Answer from the drawing. Dimensions are ordinates in mm from the lowest x, y and z of the part. Give positions to 0.01 mm unless a question says otherwise; leave off trailing zeros. Write each loop counter-clockwise with the first axis right and the second up, starting at its lowest first coordinate (ties: lowest second). Pieces come first, ordered by that corner, then holes.
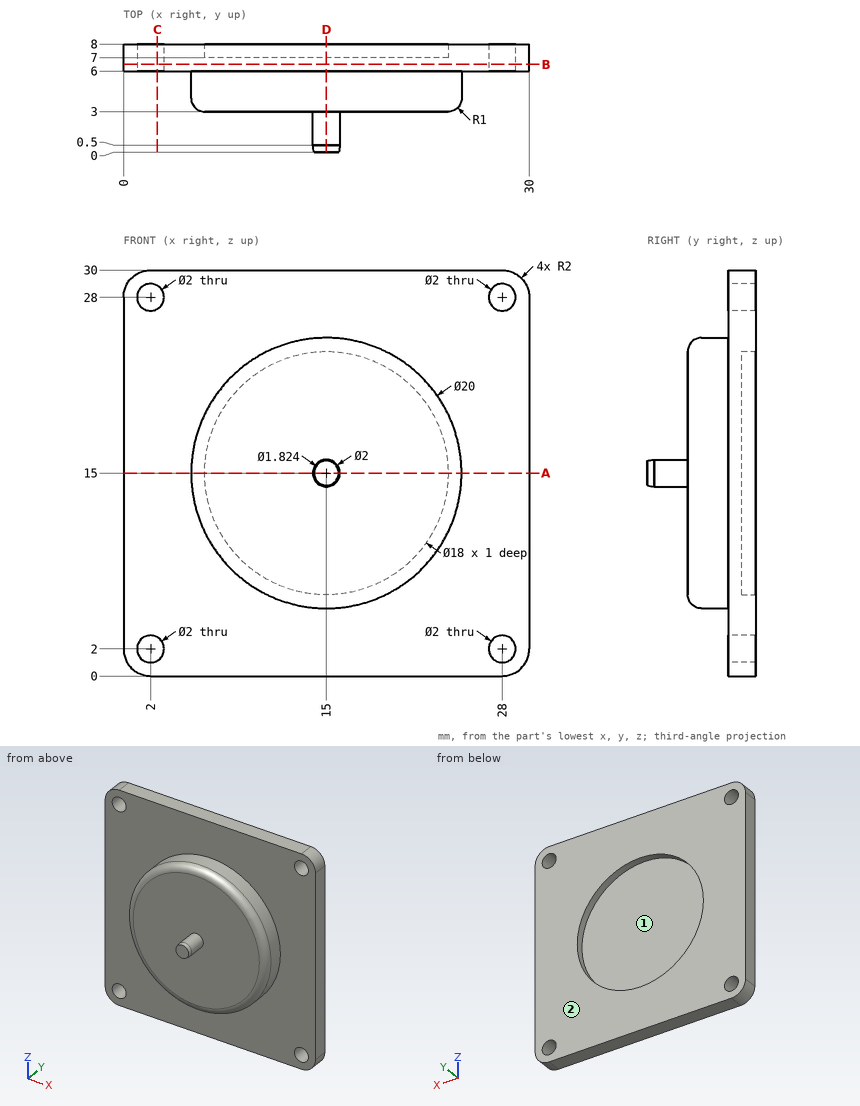
Item 1: Each of these flat-tipped pins is pushed along its axis until it touches: pin 1 Ø1.6 at (x, z) = (28, 28) entering from -Y; pin 2 Ø9 at (x, z) = (17, 15.5) entering from +Y; pin 3 Ø12 at (x, z) = (17.5, 26) entering from -Y; pin 4 Ø4 at (x, y) = (13, 3.5) entering from -Z. Where does it stop, or does it pass through?
Result set:
pin 1: passes through
pin 2: stops at y = 7
pin 3: stops at y = 3
pin 4: stops at z = 5
Item 2: Determine the mould class of the marked faces 1 and 2 for opening direction X: pulls with the +X half, pulls with the -X half, needs draft (parallel to the pull), parting line crosses it, or undercut.
Result set:
face 1: undercut
face 2: needs draft
Item 3: Section B-B (y = 6.5) is taken. Write down the section's boundary in (x, z), and give its area (3 significant figures).
Result set:
outline: (0, 2) arc R2 ccw to (2, 0) - (28, 0) arc R2 ccw to (30, 2) - (30, 28) arc R2 ccw to (28, 30) - (2, 30) arc R2 ccw to (0, 28) - close; hole circle Ø2 at (2, 2); hole circle Ø2 at (2, 28); hole circle Ø2 at (28, 2); hole circle Ø2 at (28, 28)
area: 884 mm2
Item 4: Section A-A (z = 15) is taken. Write down the section's boundary in (x, y).
Result set:
outline: (0, 6) - (5, 6) - (5, 4) arc R1 ccw to (6, 3) - (14, 3) - (14, 0.5) - (14.09, 0) - (15.91, 0) - (16, 0.5) - (16, 3) - (24, 3) arc R1 ccw to (25, 4) - (25, 6) - (30, 6) - (30, 8) - (24, 8) - (24, 7) - (6, 7) - (6, 8) - (0, 8) - close
Item 5: Section D-D (x = 15) is taken. Write down the section's boundary in (y, z).
Result set:
outline: (0, 14.09) - (0.5, 14) - (3, 14) - (3, 6) arc R1 ccw to (4, 5) - (6, 5) - (6, 0) - (8, 0) - (8, 6) - (7, 6) - (7, 24) - (8, 24) - (8, 30) - (6, 30) - (6, 25) - (4, 25) arc R1 ccw to (3, 24) - (3, 16) - (0.5, 16) - (0, 15.91) - close
Item 6: Section C-C (x = 2.5) is taken. Write down the section's boundary in (y, z).
Result set:
outline: (6, 0) - (8, 0) - (8, 1.13) - (6, 1.13) - close; (6, 2.87) - (8, 2.87) - (8, 27.13) - (6, 27.13) - close; (6, 28.87) - (8, 28.87) - (8, 30) - (6, 30) - close
Item 7: Find the intervals of material crossed by line 1 along Z through (x, y) = (28, 6.6); line 2 along X through (y, z) = (7.5, 15), in increasing order.
Result set:
line 1: z = 0 to 1, 3 to 27, 29 to 30
line 2: x = 0 to 6, 24 to 30
